```python
from build123d import *

# Parameters (mm, degrees)
TAGLIO_ESTRUSIONE1_START = -7
TAGLIO_ESTRUSIONE1_DEPTH = 7


with BuildPart() as part:
    # Schizzo2 → Rivoluzione1 (revolve)
    with BuildSketch(Plane.XY):
        with BuildLine():
            Line((-9, -21.170817104), (-9, -7.170817104))
            add(Edge.make_bspline(
                [(-9, -2.170817104), (-11.983123447, -3.356989604), (-9, -7.170817104)],
                knots=[0, 0, 0, 1, 1, 1], degree=2))
            Line((-9, -2.170817104), (-7.5, -2.170817104))
            Line((-7.5, -2.170817104), (-7.5, -29.670817104))
            Line((-7.5, -29.670817104), (-6, -29.670817104))
            Line((-6, -29.670817104), (-6, -57.170817104))
            Line((-6, -57.170817104), (-9, -57.170817104))
            Line((-9, -57.170817104), (-9, -29.170817104))
            Line((-9, -29.170817104), (-14, -29.170817104))
            Line((-14, -29.170817104), (-14, -27.170817104))
            Line((-14, -27.170817104), (-10, -27.170817104))
            Line((-10, -27.170817104), (-10, -26.170817104))
            Line((-10, -26.170817104), (-14, -26.170817104))
            Line((-14, -26.170817104), (-14, -22.170817104))
            ThreePointArc((-14, -22.170817104), (-14.5, -21.670817104), (-14, -21.170817104))
            Line((-14, -21.170817104), (-9, -21.170817104))
        make_face()
    revolve(axis=Axis((0, 18.35883479, 0), (0, -1, 0)))

    # Schizzo5 → Taglio-Estrusione1 (cut)
    with BuildSketch(Plane.XZ.offset(29.170817104).offset(TAGLIO_ESTRUSIONE1_START)):
        with BuildLine():
            Line((1.5, 15.062469538), (-1.5, 15.062469538))
            Line((-1.5, 15.062469538), (-1.5, 8.874119675))
            ThreePointArc((-1.5, 8.874119675), (0, 9), (1.5, 8.874119675))
            Line((1.5, 8.874119675), (1.5, 15.062469538))
        make_face()
        with BuildLine():
            Line((11.711434524, 9.59011418), (7.335610371, 5.214290027))
            ThreePointArc((7.335610371, 5.214290027), (6.363961031, 6.363961031), (5.214290027, 7.335610371))
            Line((5.214290027, 7.335610371), (9.59011418, 11.711434524))
            Line((9.59011418, 11.711434524), (11.711434524, 9.59011418))
        make_face()
        with BuildLine():
            Line((15.062469538, -1.5), (8.874119675, -1.5))
            ThreePointArc((8.874119675, -1.5), (9, 0), (8.874119675, 1.5))
            Line((8.874119675, 1.5), (15.062469538, 1.5))
            Line((15.062469538, 1.5), (15.062469538, -1.5))
        make_face()
        with BuildLine():
            Line((9.59011418, -11.711434524), (5.214290027, -7.335610371))
            ThreePointArc((5.214290027, -7.335610371), (6.363961031, -6.363961031), (7.335610371, -5.214290027))
            Line((7.335610371, -5.214290027), (11.711434524, -9.59011418))
            Line((11.711434524, -9.59011418), (9.59011418, -11.711434524))
        make_face()
        with BuildLine():
            Line((-1.5, -15.062469538), (-1.5, -8.874119675))
            ThreePointArc((-1.5, -8.874119675), (0, -9), (1.5, -8.874119675))
            Line((1.5, -8.874119675), (1.5, -15.062469538))
            Line((1.5, -15.062469538), (-1.5, -15.062469538))
        make_face()
        with BuildLine():
            Line((-11.711434524, -9.59011418), (-7.335610371, -5.214290027))
            ThreePointArc((-7.335610371, -5.214290027), (-6.363961031, -6.363961031), (-5.214290027, -7.335610371))
            Line((-5.214290027, -7.335610371), (-9.59011418, -11.711434524))
            Line((-9.59011418, -11.711434524), (-11.711434524, -9.59011418))
        make_face()
        with BuildLine():
            Line((-15.062469538, 1.5), (-8.874119675, 1.5))
            ThreePointArc((-8.874119675, 1.5), (-9, 0), (-8.874119675, -1.5))
            Line((-8.874119675, -1.5), (-15.062469538, -1.5))
            Line((-15.062469538, -1.5), (-15.062469538, 1.5))
        make_face()
        with BuildLine():
            Line((-9.59011418, 11.711434524), (-5.214290027, 7.335610371))
            ThreePointArc((-5.214290027, 7.335610371), (-6.363961031, 6.363961031), (-7.335610371, 5.214290027))
            Line((-7.335610371, 5.214290027), (-11.711434524, 9.59011418))
            Line((-11.711434524, 9.59011418), (-9.59011418, 11.711434524))
        make_face()
    extrude(amount=TAGLIO_ESTRUSIONE1_DEPTH, mode=Mode.SUBTRACT)


solid = part.part
```
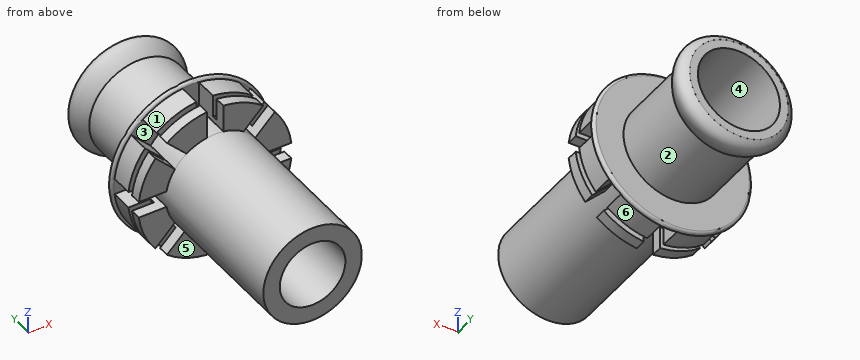
The listing builds one solid part. Answer for the finished solid, in the listing's coordinates (mm). Face numbers are marked on the shaded views. A direction names the side the tool comes from. Coordinates: 2 decimals unless noted, no trailing zeros. Loops run counter-clockwise (first coordinate to the right, second up) from the corner with the lowest first, then second, coordinate; pieces in that order, holes last. Notation, with made-up numbers: (30.25, 8) - (81.25, 8) arc R23 ccw to (81.25, 22) - close; hole circle Ø6 at (44, 49). An arc over 180 degrees is marked (long way). Use a Markdown table: item, result. Add a question column.
1) The part is cut by section B-B, the plane z = -12. State how many separate pieces and enclosed holes the cut face has, and give its area (3 significant figures).
2) The part is cut by section C-C, the plane y = -44. Give the vertices of the cut face in (x, z).
3) The mould has two halves that part along Z. Classify the marked faces 4, 5 and 6: released by +Z, released by -Z, zero draft, split by the parting line, or undercut.
4) Given pin 1 (1.7 mm diameter, centred on x = 9, z = 8.5, fed in from -Y); pin 2 (5 mm diameter, centred on x = 5.5, y = -31, fed in from -Z); pin 3 (4.5 mm diameter, centred on x = 9, z = -7.5, fed in from -Y); pin 4 (2 mm diameter, centred on y = -12, z = 10.5, fed in from -X) (3 decimals), each flat-ended and moving along its own axis, determine where each tip first touches the part or whether it passes through.
5) The part is cut by section A-A, the plane y = -17. Give the vertices of the cut face in (x, z).
6) For the marked faces 1, 2 and 3, determine the directions among +Z, -Z, +X, -X, +Y, -Y from which every point of the face is accessible in a straight line to the end or side of a thin tool.
7) Find the intervals of material crossed by line 1 (Y direction, x = -10.75, z = -8); line 2 (Z direction, x = 0, y = -40.25); line 3 (X direction, y = -20.5, z = 0), in increasing order.
Here are the results:
| question | item | result |
|---|---|---|
| 1 | separate pieces | 3 |
| 1 | enclosed holes | 0 |
| 1 | area | 84.4 mm^2 |
| 2 | outline | circle Ø18 at (0, 0); hole circle Ø12 at (0, 0) |
| 3 | face 4 | undercut |
| 3 | face 5 | zero draft |
| 3 | face 6 | released by -Z |
| 4 | pin 1 | stops at y = -22.17 |
| 4 | pin 2 | stops at z = -13.48 |
| 4 | pin 3 | stops at y = -29.17 |
| 4 | pin 4 | passes through |
| 5 | outline | circle Ø18 at (0, 0); hole circle Ø15 at (0, 0) |
| 6 | face 1 | +Z, -X, -Y |
| 6 | face 2 | none |
| 6 | face 3 | -Y |
| 7 | line 1 | y = -29.17 to -27.17, -26.17 to -21.17 |
| 7 | line 2 | z = -9 to -6, 6 to 9 |
| 7 | line 3 | x = -9 to -7.5, 7.5 to 9 |
